Can you work these out from the model? Positions are in its coordinate system, mm. Round coordinates to 2 decimals unless told otherwise and drop trailing zeros. Write each loop counter-clockwise with the first axis right and the second up, starting at its lowest first coordinate (ties: lowest second). Pieces come first, ordered by that corner, then holes. Notation, with made-up numbers: M -1.75,84.25 L 55.25,84.25 A29 cw 55.25,107.25 Z; hole C 48.5,89.25 d10. An arc over 180 degrees is marked long. Answer as a JSON object with one key per item and string values. Group by question number.
1) Please list where these lines run through material, in increasing order: L1, parallel to Z at x = 274, y = 64.5; L2, parallel to Z at x = 252, y = 95. Write a range as [from, to].
2) Suppose I cut it at B-B, the plane z = 8. Write out the boundary of the cut face in (x, y), and give its area (3 significant figures).
3) If we mould it in two halves opening along Y, with no side actions, what happens to faces 1 (the flat face through (207, 274, 0)), 2 (the flat face through (49.757, 68.114, 7.465))? For each: +Y half, -Y half, draft (parallel to the pull), parting line (faces both ways), or undercut.
4) I'm going to push a flat-ended pin straight in: pin 1 Ø19 at (x, y) = (140, 455.5) entering from +Z. Where does the tip first touch, or does it pass through?
from build123d import *
from OCP.BRepFilletAPI import BRepFilletAPI_MakeChamfer

# Parameters (mm, degrees)
ESQUISSE1_W             = 420
ESQUISSE1_H             = 540
BOSS_EXTRU_1_DEPTH      = 10
ENL_V_MAT_EXTRU_1_DEPTH = 5
CHANFREIN1_SIZE         = 5
CHANFREIN1_SIZE_2       = 13.737387097


with BuildPart() as part:
    # Esquisse1 → Boss.-Extru.1 (new body)
    with BuildSketch(Plane.XY):
        with Locations((210, 270)):
            Rectangle(ESQUISSE1_W, ESQUISSE1_H)
    extrude(amount=BOSS_EXTRU_1_DEPTH)

    # Esquisse2 → Enlèv. mat.-Extru.1 (cut)
    with BuildSketch(Plane.XY.offset(10)):
        Polygon((300, 100), (120, 100), (70, 140), (30, 140), (30, 75), (61.25, 50), (358.75, 50), (390, 75), (390, 140), (350, 140), align=None)
        Polygon((30, 465), (61.25, 490), (358.75, 490), (390, 465), (390, 400), (350, 400), (300, 440), (120, 440), (70, 400), (30, 400), align=None)
    extrude(amount=-ENL_V_MAT_EXTRU_1_DEPTH, mode=Mode.SUBTRACT)

    # Chanfrein1
    chanfrein1_edges_1 = [part.edges().sort_by_distance(p)[0] for p in [
        (390, 107.5, 5),
    ]]
    chanfrein1_side_1 = [part.faces().sort_by_distance(p)[0] for p in [
        (390, 107.5, 5.1),
    ]]
    chanfrein1_edges_2 = [part.edges().sort_by_distance(p)[0] for p in [
        (374.375, 62.5, 5),
    ]]
    chanfrein1_side_2 = [part.faces().sort_by_distance(p)[0] for p in [
        (374.375, 62.5, 5.1),
    ]]
    chanfrein1_edges_3 = [part.edges().sort_by_distance(p)[0] for p in [
        (210, 50, 5),
    ]]
    chanfrein1_side_3 = [part.faces().sort_by_distance(p)[0] for p in [
        (210, 50, 5.1),
    ]]
    chanfrein1_edges_4 = [part.edges().sort_by_distance(p)[0] for p in [
        (45.625, 62.5, 5),
    ]]
    chanfrein1_side_4 = [part.faces().sort_by_distance(p)[0] for p in [
        (45.625, 62.5, 5.1),
    ]]
    chanfrein1_edges_5 = [part.edges().sort_by_distance(p)[0] for p in [
        (30, 107.5, 5),
    ]]
    chanfrein1_side_5 = [part.faces().sort_by_distance(p)[0] for p in [
        (30, 107.5, 5.1),
    ]]
    chanfrein1_edges_6 = [part.edges().sort_by_distance(p)[0] for p in [
        (50, 140, 5),
    ]]
    chanfrein1_side_6 = [part.faces().sort_by_distance(p)[0] for p in [
        (50, 140, 5.1),
    ]]
    chanfrein1_edges_7 = [part.edges().sort_by_distance(p)[0] for p in [
        (95, 120, 5),
    ]]
    chanfrein1_side_7 = [part.faces().sort_by_distance(p)[0] for p in [
        (95, 120, 5.1),
    ]]
    chanfrein1_edges_8 = [part.edges().sort_by_distance(p)[0] for p in [
        (210, 100, 5),
    ]]
    chanfrein1_side_8 = [part.faces().sort_by_distance(p)[0] for p in [
        (210, 100, 5.1),
    ]]
    chanfrein1_edges_9 = [part.edges().sort_by_distance(p)[0] for p in [
        (325, 120, 5),
    ]]
    chanfrein1_side_9 = [part.faces().sort_by_distance(p)[0] for p in [
        (325, 120, 5.1),
    ]]
    chanfrein1_edges_10 = [part.edges().sort_by_distance(p)[0] for p in [
        (370, 140, 5),
    ]]
    chanfrein1_side_10 = [part.faces().sort_by_distance(p)[0] for p in [
        (370, 140, 5.1),
    ]]
    chanfrein1_edges_11 = [part.edges().sort_by_distance(p)[0] for p in [
        (45.625, 477.5, 5),
    ]]
    chanfrein1_side_11 = [part.faces().sort_by_distance(p)[0] for p in [
        (45.625, 477.5, 5.1),
    ]]
    chanfrein1_edges_12 = [part.edges().sort_by_distance(p)[0] for p in [
        (210, 490, 5),
    ]]
    chanfrein1_side_12 = [part.faces().sort_by_distance(p)[0] for p in [
        (210, 490, 5.1),
    ]]
    chanfrein1_edges_13 = [part.edges().sort_by_distance(p)[0] for p in [
        (374.375, 477.5, 5),
    ]]
    chanfrein1_side_13 = [part.faces().sort_by_distance(p)[0] for p in [
        (374.375, 477.5, 5.1),
    ]]
    chanfrein1_edges_14 = [part.edges().sort_by_distance(p)[0] for p in [
        (390, 432.5, 5),
    ]]
    chanfrein1_side_14 = [part.faces().sort_by_distance(p)[0] for p in [
        (390, 432.5, 5.1),
    ]]
    chanfrein1_edges_15 = [part.edges().sort_by_distance(p)[0] for p in [
        (370, 400, 5),
    ]]
    chanfrein1_side_15 = [part.faces().sort_by_distance(p)[0] for p in [
        (370, 400, 5.1),
    ]]
    chanfrein1_edges_16 = [part.edges().sort_by_distance(p)[0] for p in [
        (325, 420, 5),
    ]]
    chanfrein1_side_16 = [part.faces().sort_by_distance(p)[0] for p in [
        (325, 420, 5.1),
    ]]
    chanfrein1_edges_17 = [part.edges().sort_by_distance(p)[0] for p in [
        (210, 440, 5),
    ]]
    chanfrein1_side_17 = [part.faces().sort_by_distance(p)[0] for p in [
        (210, 440, 5.1),
    ]]
    chanfrein1_edges_18 = [part.edges().sort_by_distance(p)[0] for p in [
        (95, 420, 5),
    ]]
    chanfrein1_side_18 = [part.faces().sort_by_distance(p)[0] for p in [
        (95, 420, 5.1),
    ]]
    chanfrein1_edges_19 = [part.edges().sort_by_distance(p)[0] for p in [
        (50, 400, 5),
    ]]
    chanfrein1_side_19 = [part.faces().sort_by_distance(p)[0] for p in [
        (50, 400, 5.1),
    ]]
    chanfrein1_edges_20 = [part.edges().sort_by_distance(p)[0] for p in [
        (30, 432.5, 5),
    ]]
    chanfrein1_side_20 = [part.faces().sort_by_distance(p)[0] for p in [
        (30, 432.5, 5.1),
    ]]
    chanfrein1 = BRepFilletAPI_MakeChamfer(part.part.solid().wrapped)
    for e in chanfrein1_edges_1:
        chanfrein1.Add(CHANFREIN1_SIZE - 0.0001, CHANFREIN1_SIZE_2 - 0.0001, e.wrapped, chanfrein1_side_1[0].wrapped)
    for e in chanfrein1_edges_2:
        chanfrein1.Add(CHANFREIN1_SIZE - 0.0001, CHANFREIN1_SIZE_2 - 0.0001, e.wrapped, chanfrein1_side_2[0].wrapped)
    for e in chanfrein1_edges_3:
        chanfrein1.Add(CHANFREIN1_SIZE - 0.0001, CHANFREIN1_SIZE_2 - 0.0001, e.wrapped, chanfrein1_side_3[0].wrapped)
    for e in chanfrein1_edges_4:
        chanfrein1.Add(CHANFREIN1_SIZE - 0.0001, CHANFREIN1_SIZE_2 - 0.0001, e.wrapped, chanfrein1_side_4[0].wrapped)
    for e in chanfrein1_edges_5:
        chanfrein1.Add(CHANFREIN1_SIZE - 0.0001, CHANFREIN1_SIZE_2 - 0.0001, e.wrapped, chanfrein1_side_5[0].wrapped)
    for e in chanfrein1_edges_6:
        chanfrein1.Add(CHANFREIN1_SIZE - 0.0001, CHANFREIN1_SIZE_2 - 0.0001, e.wrapped, chanfrein1_side_6[0].wrapped)
    for e in chanfrein1_edges_7:
        chanfrein1.Add(CHANFREIN1_SIZE - 0.0001, CHANFREIN1_SIZE_2 - 0.0001, e.wrapped, chanfrein1_side_7[0].wrapped)
    for e in chanfrein1_edges_8:
        chanfrein1.Add(CHANFREIN1_SIZE - 0.0001, CHANFREIN1_SIZE_2 - 0.0001, e.wrapped, chanfrein1_side_8[0].wrapped)
    for e in chanfrein1_edges_9:
        chanfrein1.Add(CHANFREIN1_SIZE - 0.0001, CHANFREIN1_SIZE_2 - 0.0001, e.wrapped, chanfrein1_side_9[0].wrapped)
    for e in chanfrein1_edges_10:
        chanfrein1.Add(CHANFREIN1_SIZE - 0.0001, CHANFREIN1_SIZE_2 - 0.0001, e.wrapped, chanfrein1_side_10[0].wrapped)
    for e in chanfrein1_edges_11:
        chanfrein1.Add(CHANFREIN1_SIZE - 0.0001, CHANFREIN1_SIZE_2 - 0.0001, e.wrapped, chanfrein1_side_11[0].wrapped)
    for e in chanfrein1_edges_12:
        chanfrein1.Add(CHANFREIN1_SIZE - 0.0001, CHANFREIN1_SIZE_2 - 0.0001, e.wrapped, chanfrein1_side_12[0].wrapped)
    for e in chanfrein1_edges_13:
        chanfrein1.Add(CHANFREIN1_SIZE - 0.0001, CHANFREIN1_SIZE_2 - 0.0001, e.wrapped, chanfrein1_side_13[0].wrapped)
    for e in chanfrein1_edges_14:
        chanfrein1.Add(CHANFREIN1_SIZE - 0.0001, CHANFREIN1_SIZE_2 - 0.0001, e.wrapped, chanfrein1_side_14[0].wrapped)
    for e in chanfrein1_edges_15:
        chanfrein1.Add(CHANFREIN1_SIZE - 0.0001, CHANFREIN1_SIZE_2 - 0.0001, e.wrapped, chanfrein1_side_15[0].wrapped)
    for e in chanfrein1_edges_16:
        chanfrein1.Add(CHANFREIN1_SIZE - 0.0001, CHANFREIN1_SIZE_2 - 0.0001, e.wrapped, chanfrein1_side_16[0].wrapped)
    for e in chanfrein1_edges_17:
        chanfrein1.Add(CHANFREIN1_SIZE - 0.0001, CHANFREIN1_SIZE_2 - 0.0001, e.wrapped, chanfrein1_side_17[0].wrapped)
    for e in chanfrein1_edges_18:
        chanfrein1.Add(CHANFREIN1_SIZE - 0.0001, CHANFREIN1_SIZE_2 - 0.0001, e.wrapped, chanfrein1_side_18[0].wrapped)
    for e in chanfrein1_edges_19:
        chanfrein1.Add(CHANFREIN1_SIZE - 0.0001, CHANFREIN1_SIZE_2 - 0.0001, e.wrapped, chanfrein1_side_19[0].wrapped)
    for e in chanfrein1_edges_20:
        chanfrein1.Add(CHANFREIN1_SIZE - 0.0001, CHANFREIN1_SIZE_2 - 0.0001, e.wrapped, chanfrein1_side_20[0].wrapped)
    add(Compound.cast(chanfrein1.Shape()), mode=Mode.REPLACE)  # a hair under: the kernel refuses the full size


solid = part.part
Results:
{
 "1": {"L1": "[0, 5]", "L2": "[0, 8.18]"},
 "2": {"outline": "M 0,0 L 420,0 L 420,540 L 0,540 Z; hole M 35.49,77.64 L 63.18,55.49 L 356.82,55.49 L 384.51,77.64 L 384.51,134.51 L 351.93,134.51 L 301.93,94.51 L 118.07,94.51 L 68.07,134.51 L 35.49,134.51 Z; hole M 35.49,405.49 L 68.07,405.49 L 118.07,445.49 L 301.93,445.49 L 351.93,405.49 L 384.51,405.49 L 384.51,462.36 L 356.82,484.51 L 63.18,484.51 L 35.49,462.36 Z", "area": "192,000 mm^2"},
 "3": {"face 1": "draft", "face 2": "undercut"},
 "4": {"pin 1": "z = 7.82"}
}
